Solid Edge part; units mm, degrees
sketch "Sketch1" plane through (0, 0, 53.9958) normal (0, 0, 1) x (1, 0, 0)
  line L0 (-103.5004, 98.9905) -> (28.9996, 98.9996)
  line L1 (29.0004, 88.9996) -> (-103.4997, 88.9905)
  arc A0 (-103.5004, 98.9905) -> (-103.4997, 88.9905) centre (-103.5, 93.9905) ccw
  arc A1 (28.9996, 98.9996) -> (29.0004, 88.9996) centre (29, 93.9996) cw
  circle A2 centre (-103.5, 93.9905) radius 0.8
extrude "Protrusion1" add sketch "Sketch1" against normal blind 4
sketch "Sketch2" plane through (-37.25, 93.9951, 53.9958) normal (0, 0, 1) x (1, 0.0001, 0)
  circle A0 centre (66.25, 0) radius 5
  circle A1 centre (66.25, 0) radius 0.8
extrude "ExtrudedProtrusion_5" add sketch "Sketch2" along normal blind 5
Source: CAD feature listing. Evaluate the final solid. Frame: model axes, mm. A direction names the side the tool comes from. Round coordinates to 2 decimals unless told otherwise and drop trailing zeros. Loops run counter-clockwise (first coordinate to the right, second up) from the corner with the lowest first, then second, coordinate; pieces in that order, holes last. Notation, with made-up numbers: (6.25, -39.75) -> (37.25, -39.75) arc R20 cw to (37.25, -6.75) -> close; hole circle Ø3 at (-15.5, 6.25). An arc over 180 degrees is marked (long way). Answer as a JSON object with one key per item and string values. Group by question number.
Q1. Access query for faces 1 (the flat face through (-36, 94, 49.996)), 2 (the cylindrical face through (27.916, 98.876, 56.461)). Directions: +Z, -Z, +X, -X, +Y, -Y. A direction counts if a zero-diameter tool reaches every point of the face in a straight line with its end or side. Return the directions, or none.
Q2. Ray query, line 1 (Y direction, x = -103.5, z = 51); line 2 (Y direction, x = 14, z = 51.5); line 3 (Z direction, x = -44, y = 96.5). Return the intervals inside material, ascending. Write a range as from..to.
Q3. Mould query, pull axis X, two halves, no side actions, for faces 3 (the flat face through (29, 93, 58.996)), 4 (the cylindrical face through (-108.5, 94.1, 52)), 5 (the cylindrical face through (34, 94, 52)). Classes: pulls with the +X half, pulls with the -X half, needs draft (parallel to the pull), parting line crosses it, or undercut.
Q4. Section query B-B (x = -94). Output: boundary loops of the cut face in (y, z).
Q5. Section query A-A (z = 56.25). Output: boundary loops of the cut face in (x, y).
Q6. Contact query for flat-ended pins moving along their axis: P1, Ø5, axis at x = -58, y = 92.5, coming from the +Z side; P2, Ø2, axis at x = -24, z = 51.5, coming from the +Y side; P3, Ø5, axis at y = 90, z = 53.5, coming from the +X side. Output: stop coordinate, or through.
Completed:
{
 "1": {"face 1": "-Z, +X, -X, +Y, -Y", "face 2": "+Z"},
 "2": {"line 1": "88.99..93.19, 94.79..98.99", "line 2": "89..99", "line 3": "50..54"},
 "3": {"face 3": "needs draft", "face 4": "pulls with the -X half", "face 5": "pulls with the +X half"},
 "4": {"outline": "(88.99, 50) -> (98.99, 50) -> (98.99, 54) -> (88.99, 54) -> close"},
 "5": {"outline": "circle Ø10 at (29, 94); hole circle Ø1.6 at (29, 94)"},
 "6": {"P1": "z = 54", "P2": "y = 99", "P3": "x = 33.77"}
}
